Input: part model. Units: mm. Frame: model coordinates. Face numbers are marked on the shaded views. A direction names the side the tool comes from. Coordinates: 2 decimals unless noted, no trailing zeros. Loops run counter-clockwise (first coordinate to the right, second up) from the corner with the lowest first, then second, coordinate; pieces in that order, holes last. Notation, with made-up numbers: (48.25, 57) - (56.25, 57) arc R11 cw to (56.25, 72) - close; hole circle Ø9 at (67.25, 28). An arc over 180 degrees is marked (long way). Use a Markdown table: item, result. Add a question column.
1. Contact query for flat-ended pins moving along their axis: P1, Ø1, axis at y = 36, z = 130, coming from the -X side; P2, Ø1.5, axis at x = -4, z = 130.5, coming from the -Y side; P3, Ø1.2, axis at x = -3, y = 38, coming from the -Z side. Output: stop coordinate, or through.
2. Access query for the marked faces 1, 2 and 3. Directions: +Z, -Z, +X, -X, +Y, -Y. A direction counts if a zero-diameter tool reaches every point of the face in a straight line with its end or side. Return the directions, or none.
3. Ray query, L1, parallel to X at y = 35.55, z = 122.5; L2, parallel to Z at x = -1.7, y = 35.3; L3, parallel to Y at x = -3.8, z = 122.75. Return the intervals inside material, ascending. Write a range as [from, to].
4. Draft query along Y for the marked faces 4, 5 and 6. Return one class per face: released by +Y, released by -Y, zero draft, split by the parting line, or undercut.
5. Section query A-A on y = 38.95. Return the cut outline in (x, z).
6. Section query C-C on z = 131.5. Return the cut outline in (x, y).
7. Section query B-B on x = -0.75. Return the cut outline in (y, z), then the cut area to 3 significant figures.
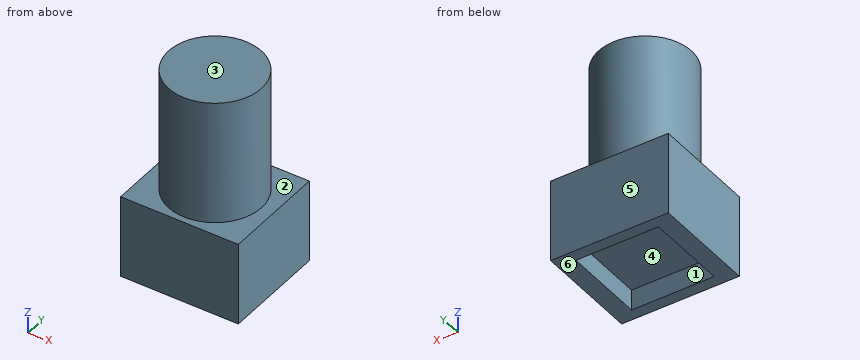
```python
from build123d import *

# Parameters (mm, degrees)
SCHIZZO1_W                   = 5.699999879
SCHIZZO1_H                   = 5.099999898
ESTRUSIONE_ESTRUSIONE1_DEPTH = 4
SCHIZZO2_W                   = 4
SCHIZZO2_H                   = 4
TAGLIO_ESTRUSIONE1_DEPTH     = 1
SCHIZZO3_R                   = 2.25
ESTRUSIONE_ESTRUSIONE2_DEPTH = 6


with BuildPart() as part:
    # Schizzo1 → Estrusione-Estrusione1 (new body)
    with BuildSketch(Plane(origin=(0, 0, 126.00326253), x_dir=(-1, 0, 0), z_dir=(0, 0, -1))):
        with Locations((2.391212038, 37.24404717)):
            Rectangle(SCHIZZO1_W, SCHIZZO1_H)
    extrude(amount=ESTRUSIONE_ESTRUSIONE1_DEPTH)

    # Schizzo2 → Taglio-Estrusione1 (cut)
    with BuildSketch(Plane(origin=(0, 0, 122.00326253), x_dir=(-1, 0, 0), z_dir=(0, 0, -1))):
        with Locations((2.391212098, 37.244047119)):
            Rectangle(SCHIZZO2_W, SCHIZZO2_H)
    extrude(amount=-TAGLIO_ESTRUSIONE1_DEPTH, mode=Mode.SUBTRACT)

    # Schizzo3 → Estrusione-Estrusione2 (add)
    with BuildSketch(Plane.XY.offset(126.00326253)):
        with Locations((-2.391212038, 37.24404717)):
            Circle(SCHIZZO3_R)
    extrude(amount=ESTRUSIONE_ESTRUSIONE2_DEPTH)


solid = part.part
```
Resolved:
| question | item | result |
|---|---|---|
| 1 | P1 | x = -4.51 |
| 1 | P2 | y = 35.16 |
| 1 | P3 | z = 123 |
| 2 | face 1 | -Z |
| 2 | face 2 | +Z |
| 2 | face 3 | +Z, +X, -X, +Y, -Y |
| 3 | L1 | [-5.24, -4.39], [-0.39, 0.46] |
| 3 | L2 | [123, 132] |
| 3 | L3 | [34.69, 35.24], [39.24, 39.79] |
| 4 | face 4 | undercut |
| 4 | face 5 | released by +Y |
| 4 | face 6 | zero draft |
| 5 | outline | (-5.24, 122) - (-4.39, 122) - (-4.39, 123) - (-0.39, 123) - (-0.39, 122) - (0.46, 122) - (0.46, 126) - (-0.92, 126) - (-0.92, 132) - (-3.86, 132) - (-3.86, 126) - (-5.24, 126) - close |
| 6 | outline | circle Ø4.5 at (-2.39, 37.24) |
| 7 | outline | (34.69, 122) - (35.24, 122) - (35.24, 123) - (39.24, 123) - (39.24, 122) - (39.79, 122) - (39.79, 126) - (38.78, 126) - (38.78, 132) - (35.7, 132) - (35.7, 126) - (34.69, 126) - close |
| 7 | area | 34.9 mm² |
